Input: part model. Units: mm. Frame: model coordinates. Round coordinates to 2 decimals unless told otherwise and drop trailing zeros. Loops run counter-clockwise (first coordinate to the right, second up) from the corner with the lowest first, then second, coordinate; pieces in that order, holes last. Notation, with made-up numbers: (77, 43.25) -> (135, 43.25) arc R22 ccw to (135, 71.25) -> close; hole circle Ø3 at (-15, 80). An arc over 180 degrees is marked (long way). Answer in a Markdown table with one row per item. Add a question column.
Q1. Section B-B, the plane z = 217.5. Output: boundary loops of the cut face in (x, y), and give its area (3 significant figures).
Q2. Pin query (flat end, axial travel): pin 1 (2.5 mm diameter, centred on y = 5.7, z = 89.35, fed in from +X). Return the tip coordinate at first contact, or that it passes through.
Q3. Ray query, L1, parallel to Z at x = 5.7, y = 2.5; L2, parallel to X at y = 5.7, z = 15.5. Return the intervals inside material, ascending. Write a range as from..to.
Q4. Section A-A, the plane x = 9.5. Give the number of separate pieces and of enclosed holes in the cut face, and give its area (3 significant figures).
```python
from build123d import *

# Parameters (mm, degrees)
SKETCH_W        = 11.4
SKETCH_H        = 11.4
SKETCH_R        = 1.5
PAD_DEPTH       = 275.2
SKETCH001_R     = 1.5
POCKET_DEPTH    = 11.401
SKETCH002_R     = 1.5
POCKET001_DEPTH = 11.401


with BuildPart() as part:
    # Sketch → Pad (new body)
    with BuildSketch(Plane.XY):
        with Locations((5.7, 5.7)):
            Rectangle(SKETCH_W, SKETCH_H)
        with Locations((5.7, 5.7)):
            Circle(SKETCH_R, mode=Mode.SUBTRACT)
    extrude(amount=PAD_DEPTH)

    # Sketch001 → Pocket (cut, through all)
    with BuildSketch(Plane.YZ.offset(11.4)):
        with Locations((5.7, 142.35)):
            Circle(SKETCH001_R)
        with Locations((5.7, 134.35)):
            Circle(SKETCH001_R)
        with Locations((5.7, 19)):
            Circle(SKETCH001_R)
        with Locations((5.7, 11)):
            Circle(SKETCH001_R)
        with Locations((5.7, 89.35)):
            Circle(SKETCH001_R)
        with Locations((5.7, 81.35)):
            Circle(SKETCH001_R)
        with Locations((5.7, 264.2)):
            Circle(SKETCH001_R)
        with Locations((5.7, 256.2)):
            Circle(SKETCH001_R)
    extrude(amount=-POCKET_DEPTH, mode=Mode.SUBTRACT)

    # Sketch002 → Pocket001 (cut, through all)
    with BuildSketch(Plane(origin=(0, 11.4, 0), x_dir=(-1, 0, 0), z_dir=(0, 1, 0))):
        with Locations((-5.7, 60)):
            Circle(SKETCH002_R)
        with Locations((-5.7, 97)):
            Circle(SKETCH002_R)
        with Locations((-5.7, 134)):
            Circle(SKETCH002_R)
    extrude(amount=-POCKET001_DEPTH, mode=Mode.SUBTRACT)


solid = part.part
```
Answer block:
| question | item | result |
|---|---|---|
| 1 | outline | (0, 0) -> (11.4, 0) -> (11.4, 11.4) -> (0, 11.4) -> close; hole circle Ø3 at (5.7, 5.7) |
| 1 | area | 123 mm^2 |
| 2 | pin 1 | through |
| 3 | L1 | 0..58.5, 61.5..95.5, 98.5..132.5, 135.5..275.2 |
| 3 | L2 | 0..4.2, 7.2..11.4 |
| 4 | separate pieces | 1 |
| 4 | enclosed holes | 8 |
| 4 | area | 3,080 mm^2 |
